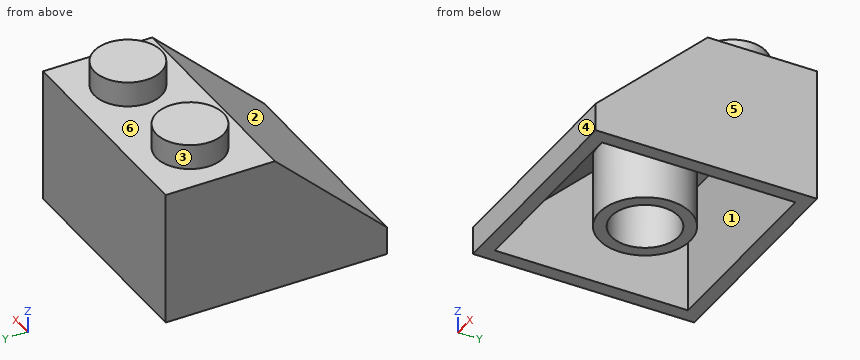
from build123d import *

# Parameters (mm, degrees)
F1_DEPTH = 7.9
F2_R     = 2.4
F3_DEPTH = 1.8
F4_T     = -1
F5_R     = 3.255
F5_R_2   = 2.4


with BuildPart() as f1:
    # F0 (on Right) → F1 (new body, symmetric)
    with BuildSketch(Plane.YZ):
        Polygon((-15.8, 0), (0, 0), (0, 9.6), (-7.8, 9.6), (-15.8, 2), align=None)
    extrude(amount=F1_DEPTH, both=True)

    # F2 (on face) → F3 (join)
    with BuildSketch(Plane.XY.offset(9.6)):
        with Locations((-4, -3.9)):
            Circle(F2_R)
        with Locations((4, -3.9)):
            Circle(F2_R)
    extrude(amount=F3_DEPTH)

    # F4
    f4_openings = [f1.faces().sort_by_distance(p)[0] for p in [
        (0, -7.9, 0),
    ]]
    offset(amount=F4_T, openings=f4_openings, kind=Kind.INTERSECTION)

    # F5 (on face) → F6 (join, up to the next surface of F1)
    with BuildSketch(Plane(origin=(0, 0, 0), x_dir=(1, 0, 0), z_dir=(0, 0, -1))):
        with Locations((0, 7.9)):
            Circle(F5_R)
        with Locations((0, 7.9)):
            Circle(F5_R_2, mode=Mode.SUBTRACT)
    extrude(until=Until.NEXT, dir=(0, 0, 1))


solid = f1.part
The listing builds one solid part. Answer for the finished solid, in the listing's coordinates (mm). Face numbers are marked on the shaded views. A direction names the side the tool comes from. Coordinates: 2 decimals unless noted, no trailing zeros. Loops run counter-clockwise (first coordinate to the right, second up) from the corner with the lowest first, then second, coordinate; pieces in that order, holes last. Notation, with made-up numbers: (47.5, -7) -> (61.5, -7) arc R17 ccw to (61.5, 9) -> close; hole circle Ø8 at (35.5, 60). An arc over 180 degrees is marked (long way). Answer in a Markdown table with one row per item. Add a question column.
1. The part is cut by section D-D, the plane y = -5.75. Write down the section's boundary in (x, z), then the cut area to 3 significant figures.
2. Flat-ended cylindrical pins translate along their axes: P1, Ø3, axis at x = 4.5, z = 9.5, coming from the +Y side; P2, Ø6, axis at x = 0, y = -7.9, coming from the +Z side; P3, Ø5, axis at x = -3.5, z = 6, coming from the -Y side; P4, Ø2, axis at x = 4, y = -3.9, coming from the -Z side. Find the tip coordinate at first contact, or state that the pin passes through.
3. The part is cut by section A-A, the plane z = 1.25. Write down the section's boundary in (x, y) (3 decimals), then the cut area to 3 significant figures.
4. Consider line 1 (X direction, y = -7.9, z = 2.5) (3 decimals); line 2 (X direction, y = -3.9, z = 9.05); line 3 (Y direction, x = 0.25, z = 4). Determine where each line is inside the solid, lowest interval first. Write a range as [from, to].
5. Determine the mould class of the marked faces 4, 5 and 6 for opening direction X: +X half, -X half, draft (parallel to the pull), parting line (faces both ways), or undercut.
6. The part is cut by section C-C, the plane z = 4. Write down the section's boundary in (x, y) (3 decimals), then the cut area to 3 significant figures.
7. The part is cut by section B-B, the plane x = -4. Write down the section's boundary in (y, z), then the cut area to 3 significant figures.
8. For the marked faces 1, 2 and 3, determine the directions among +Z, -Z, +X, -X, +Y, -Y from which every point of the face is accessible in a straight line to the end or side of a thin tool.
Answer below:
| question | item | result |
|---|---|---|
| 1 | outline | (-7.9, 0) -> (-6.9, 0) -> (-6.9, 8.6) -> (-2.44, 8.6) -> (-2.44, 0) -> (-1.07, 0) -> (-1.07, 8.6) -> (1.07, 8.6) -> (1.07, 0) -> (2.44, 0) -> (2.44, 8.6) -> (6.9, 8.6) -> (6.9, 0) -> (7.9, 0) -> (7.9, 9.6) -> (5.53, 9.6) -> (5.53, 11.4) -> (2.47, 11.4) -> (2.47, 9.6) -> (-2.47, 9.6) -> (-2.47, 11.4) -> (-5.53, 11.4) -> (-5.53, 9.6) -> (-7.9, 9.6) -> close |
| 1 | area | 67.7 mm2 |
| 2 | P1 | y = 0 |
| 2 | P2 | z = 9.6 |
| 2 | P3 | y = -14.22 |
| 2 | P4 | z = 10.4 |
| 3 | outline | (-7.9, -15.8) -> (7.9, -15.8) -> (7.9, 0) -> (-7.9, 0) -> close; circle Ø6.51 at (0, -7.9); hole (-6.9, -14.8) -> (6.9, -14.8) -> (6.9, -1) -> (-6.9, -1) -> close; hole circle Ø4.8 at (0, -7.9) |
| 3 | area | 74.4 mm2 |
| 4 | line 1 | [-7.9, -6.9], [-3.255, -2.4], [2.4, 3.255], [6.9, 7.9] |
| 4 | line 2 | [-7.9, -5.4], [-2.6, 2.6], [5.4, 7.9] |
| 4 | line 3 | [-13.69, -12.24], [-11.15, -10.29], [-5.51, -4.65], [-1, 0] |
| 5 | face 4 | draft |
| 5 | face 5 | +X half |
| 5 | face 6 | undercut |
| 6 | outline | (-7.9, -13.695) -> (7.9, -13.695) -> (7.9, 0) -> (-7.9, 0) -> close; circle Ø6.51 at (0, -7.9); hole (-6.9, -12.243) -> (6.9, -12.243) -> (6.9, -1) -> (-6.9, -1) -> close; hole circle Ø4.8 at (0, -7.9) |
| 6 | area | 76.4 mm2 |
| 7 | outline | (-15.8, 0) -> (-14.8, 0) -> (-14.8, 1.57) -> (-7.4, 8.6) -> (-5.3, 8.6) -> (-5.3, 10.4) -> (-2.5, 10.4) -> (-2.5, 8.6) -> (-1, 8.6) -> (-1, 0) -> (0, 0) -> (0, 9.6) -> (-1.5, 9.6) -> (-1.5, 11.4) -> (-6.3, 11.4) -> (-6.3, 9.6) -> (-7.8, 9.6) -> (-15.8, 2) -> close |
| 7 | area | 32.2 mm2 |
| 8 | face 1 | -Z |
| 8 | face 2 | +Z, +X, -X, -Y |
| 8 | face 3 | +Z |
